The drawing under review shows one solid part. Ordinate dimensions are in mm from its lowest x, y, z. A direction names the side the tool comes from. Round coordinates to 2 decimals unless told otherwise and drop trailing zeros. One line per question, with ' | ' between items. Start each with the question number.
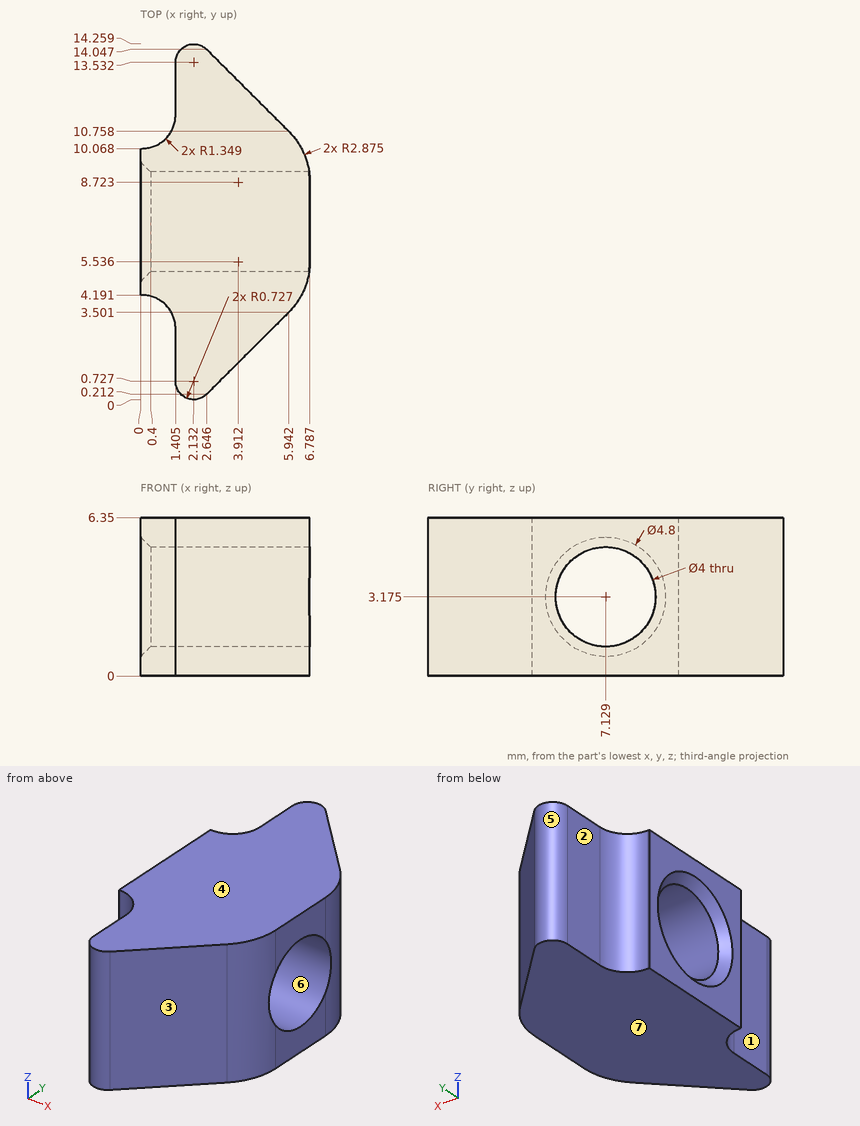
1. Clearance check with flat-ended pins moving along their axes: P1, Ø2.5, axis at y = 2, z = 4.5, coming from the -X side; P2, Ø2.5, axis at y = 12.5, z = 2, coming from the -X side (1 decimal); P3, Ø3, axis at x = 5, z = 2.5, coming from the +Y side (1 decimal); P4, Ø2, axis at y = 8.5, z = 3, coming from the +X side. State where each tip first meets the part, or that it passes through.
2. Wall thickness on line 1 along Z through (x, y) = (4, 7.5); line 2 along Y through (x, z) = (3.25, 2.25) (1 decimal); line 3 along Y through (x, z) = (1.5, 2.25) (1 decimal): over which ranges is each line inside the solid? List them lowest first. Write a range as [from, to].
3. The part is to be moulded in two halves that separate along Z. For the marked faces 4, 5, 6 and 7, say which applies: pulls with the +Z half, pulls with the -Z half, needs draft (parallel to the pull), parting line crosses it, or undercut.
4. Machinability: for the marked faces 1, 2 and 3, which of the approach directions +Z, -Z, +X, -X, +Y, -Y give a long, thin tool a straight path to every point of the face, cutting with its end or side? Answer none if there is none.
Geometry check:
1) P1: stops at x = 1.34 | P2: stops at x = 1.4 | P3: stops at y = 13.2 | P4: stops at x = 6.79
2) line 1: z = [0, 1.21], [5.14, 6.35] | line 2: y = [0.8, 5.4], [8.9, 13.4] | line 3: y = [0.4, 5.4], [8.9, 13.9]
3) face 4: pulls with the +Z half | face 5: needs draft | face 6: undercut | face 7: pulls with the -Z half
4) face 1: +Z, -Z, -X, -Y | face 2: +Z, -Z, -X, +Y | face 3: +Z, -Z, +X, -Y
